from build123d import *

# Parameters (mm, degrees)
EXTRUDE_1_DEPTH = 4.7


with BuildPart() as part:
    # 草图1 → 凸台-拉伸1 (new body)
    with BuildSketch(Plane.XY):
        Polygon((2.309401077, 4), (-2.309401077, 4), (-4.618802154, 0), (-2.309401077, -4), (2.309401077, -4), (4.618802154, 0), align=None)
    extrude(amount=EXTRUDE_1_DEPTH)

    # 草图2 → M5 螺纹孔1 (revolve, cut)
    with BuildSketch(Plane(origin=(0, 0, 4.7), x_dir=(0, -1, 0), z_dir=(1, 0, 0))):
        Polygon((0, 0), (0, 4.7), (2.525, 4.7), (2.1, 4.454626136), (2.1, 0.245373864), (2.525, 0), align=None)
    revolve(axis=Axis((0, 0, 11.05), (0, 0, -1)), mode=Mode.SUBTRACT)

    # 草图4 → 切除-旋转1 (revolve, cut)
    with BuildSketch(Plane(origin=(0, 0, 0), x_dir=(1, 0, 0), z_dir=(0, 1, 0))):
        Polygon((-4.618802154, -0.577350269), (-3.618802154, 0), (-4.618802154, 0), align=None)
        Polygon((-4.618802154, -4.7), (-3.618802154, -4.7), (-4.618802154, -4.122649731), align=None)
    revolve(axis=Axis((0, 0, 0), (0, 0, 1)), mode=Mode.SUBTRACT)


solid = part.part
Model file for the job. Use its own axes, mm. Give positions to 0.01 mm unless a question says otherwise; leave off trailing zeros. Loops run counter-clockwise (first coordinate to the right, second up) from the corner with the lowest first, then second, coordinate; pieces in that order, holes last. Notation, with made-up numbers: (22.5, 18.25) -> (42.5, 18.25) arc R12 ccw to (42.5, 29.25) -> close; hole circle Ø11 at (36, 6.25). An arc over 180 degrees is marked (long way). Use a Markdown table: item, result. Add a question column.
(1) Mould opens along Y. For faces 1 (the flat face through (0, -4, 2)), 2 (the cylindrical face through (-0.631, -2.003, 2.379)), 3 (the flat face through (-3.448, 2.028, 2.32)) say: +Y half, -Y half, draft (parallel to the pull), parting line (faces both ways), or undercut.
(2) Slice it at B-B on x = 0. List the corners of the cut face in (y, z) (3 decimals).
(3) Slice it at A-A on z = 1.3. List the corners of the cut face in (x, y), and give its area (3 significant figures).
(4) Slice it at C-C on z = 4.3. List the corners of the cut face in (x, y), and give its area (3 significant figures).
(5) Wall check: line 1 along Y through (x, z) = (0, 3.4); line 2 along Z through (x, y) = (1.5, 3.75); line 3 along Y through (x, z) = (-1.75, 4.05). Give the ranges that are in metal, low to high.
(6) Drop a flat-ended pin along its axis: pin 1 Ø2 at (y, z) = (-3, 2.5) entering from -X. Give the stop position or say it passes through.
Filled sheet:
| question | item | result |
|---|---|---|
| 1 | face 1 | -Y half |
| 1 | face 2 | undercut |
| 1 | face 3 | +Y half |
| 2 | outline | (-4, 0.22) -> (-3.619, 0) -> (-2.525, 0) -> (-2.1, 0.245) -> (-2.1, 4.455) -> (-2.525, 4.7) -> (-3.619, 4.7) -> (-4, 4.48) -> close; (2.1, 0.245) -> (2.525, 0) -> (3.619, 0) -> (4, 0.22) -> (4, 4.48) -> (3.619, 4.7) -> (2.525, 4.7) -> (2.1, 4.455) -> close |
| 3 | outline | (-4.62, 0) -> (-2.31, -4) -> (2.31, -4) -> (4.62, 0) -> (2.31, 4) -> (-2.31, 4) -> close; hole circle Ø4.2 at (0, 0) |
| 3 | area | 41.6 mm2 |
| 4 | outline | (-4.27, -0.61) -> (-2.66, -3.39) arc R4.31 ccw to (-1.61, -4) -> (1.61, -4) arc R4.31 ccw to (2.66, -3.39) -> (4.27, -0.61) arc R4.31 ccw to (4.27, 0.61) -> (2.66, 3.39) arc R4.31 ccw to (1.61, 4) -> (-1.61, 4) arc R4.31 ccw to (-2.66, 3.39) -> (-4.27, 0.61) arc R4.31 ccw to start; hole circle Ø4.2 at (0, 0) |
| 4 | area | 40.5 mm2 |
| 5 | line 1 | -4 to -2.1, 2.1 to 4 |
| 5 | line 2 | 0.24 to 4.46 |
| 5 | line 3 | -4 to -1.16, 1.16 to 4 |
| 6 | pin 1 | x = -3.46 |
